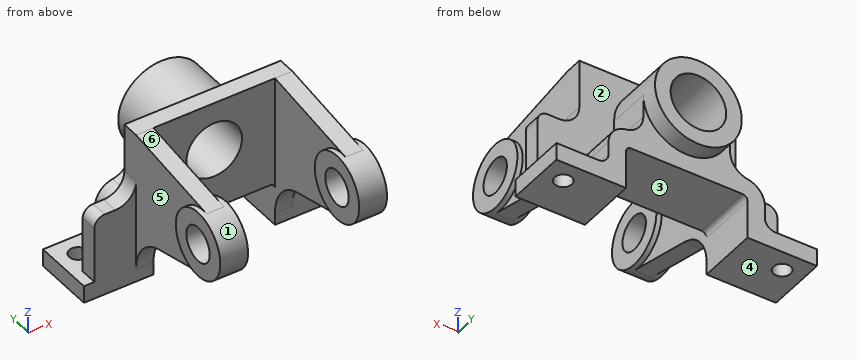
from build123d import *

# Parameters (mm, degrees)
BOSS_EXTRUDE1_DEPTH   = 10
SKETCH1_3_R           = 25
SKETCH1_3_R_2         = 16
BOSS_EXTRUDE2_DEPTH   = 45
BOSS_EXTRUDE3_DEPTH   = 35
FILLET1_R             = 12
BOSS_EXTRUDE4_DEPTH   = 10
BOSS_EXTRUDE5_START   = 3
SKETCH2_3_R           = 19
SKETCH2_3_R_2         = 10
BOSS_EXTRUDE5_DEPTH   = 16
FILLET2_R             = 25
MIRROR1_START         = -45
MIRROR1_OUTLINE_R     = 10
MIRROR1_DEPTH         = 10
MIRROR1_START_2       = -48
MIRROR1_2_OUTLINE_R   = 19
MIRROR1_2_OUTLINE_R_2 = 10
MIRROR1_2_DEPTH       = 16
SKETCH3_R             = 5
CUT_EXTRUDE1_DEPTH    = 133.483106346


# Read off the part's stored shape, not the designer's step: Mirror1
with BuildPart() as part:
    # Sketch1 → Boss-Extrude1 (new body)
    with BuildSketch(Plane(origin=(0, 0, 0), x_dir=(1, 0, 0), z_dir=(0, 1, 0))):
        with BuildLine():
            Line((-51, 50), (-69, 50))
            Line((-69, 50), (-69, 18))
            ThreePointArc((-69, 18), (-67.242640687, 13.757359313), (-63, 12))
            Line((-63, 12), (-57, 12))
            ThreePointArc((-57, 12), (-48.514718626, 8.485281374), (-45, 0))
            Line((-45, 0), (-45, -28))
            Line((-45, -28), (45, -28))
            Line((45, -28), (45, 0))
            ThreePointArc((45, 0), (48.514718626, 8.485281374), (57, 12))
            Line((57, 12), (63, 12))
            ThreePointArc((63, 12), (67.242640687, 13.757359313), (69, 18))
            Line((69, 18), (69, 50))
            Line((69, 50), (51, 50))
            ThreePointArc((51, 50), (46.757359313, 48.242640687), (45, 44))
            Line((45, 44), (45, 25))
            Line((45, 25), (37, 25))
            ThreePointArc((37, 25), (28.514718626, 21.485281374), (25, 13))
            Line((25, 13), (25, 0))
            ThreePointArc((25, 0), (0, -25), (-25, 0))
            Line((-25, 0), (-25, 13))
            ThreePointArc((-25, 13), (-28.514718626, 21.485281374), (-37, 25))
            Line((-37, 25), (-45, 25))
            Line((-45, 25), (-45, 44))
            ThreePointArc((-45, 44), (-46.757359313, 48.242640687), (-51, 50))
        make_face()
    extrude(amount=BOSS_EXTRUDE1_DEPTH)

    # Sketch1<3> → Boss-Extrude2 (add)
    with BuildSketch(Plane(origin=(0, 0, 0), x_dir=(1, 0, 0), z_dir=(0, 1, 0))):
        Circle(SKETCH1_3_R)
        with Locations(Location((0, 0, 0), (0, 0, 90))):
            Circle(SKETCH1_3_R_2, mode=Mode.SUBTRACT)
    extrude(amount=BOSS_EXTRUDE2_DEPTH)

    # Sketch1<4> → Boss-Extrude3 (add)
    with BuildSketch(Plane(origin=(0, 0, 0), x_dir=(1, 0, 0), z_dir=(0, 1, 0))):
        with BuildLine():
            Line((32, 35), (-32, 35))
            ThreePointArc((-32, 35), (-34.121320344, 35.878679656), (-35, 38))
            Line((-35, 38), (-35, 60))
            Line((-35, 60), (-75, 60))
            Line((-75, 60), (-75, 50))
            Line((-75, 50), (-69, 50))
            Line((-69, 50), (-51, 50))
            ThreePointArc((-51, 50), (-46.757359313, 48.242640687), (-45, 44))
            Line((-45, 44), (-45, 25))
            Line((-45, 25), (-37, 25))
            ThreePointArc((-37, 25), (-28.514718626, 21.485281374), (-25, 13))
            Line((-25, 13), (-25, 0))
            ThreePointArc((-25, 0), (0, 25), (25, 0))
            Line((25, 0), (25, 13))
            ThreePointArc((25, 13), (28.514718626, 21.485281374), (37, 25))
            Line((37, 25), (45, 25))
            Line((45, 25), (45, 44))
            ThreePointArc((45, 44), (46.757359313, 48.242640687), (51, 50))
            Line((51, 50), (69, 50))
            Line((69, 50), (75, 50))
            Line((75, 50), (75, 60))
            Line((75, 60), (35, 60))
            Line((35, 60), (35, 38))
            ThreePointArc((35, 38), (34.121320344, 35.878679656), (32, 35))
        make_face()
    extrude(amount=BOSS_EXTRUDE3_DEPTH)

    # Fillet1
    fillet1_edges = [part.edges().sort_by_distance(p)[0] for p in [
        (-45, 22.5, -25),
        (45, 22.5, -25),
    ]]
    fillet(fillet1_edges, radius=FILLET1_R)

    # Sketch2 → Boss-Extrude4 (add)
    with BuildSketch(Plane(origin=(45, 0, 0), x_dir=(0, 0, -1), z_dir=(1, 0, 0))):
        with BuildLine():
            Line((0, 0), (-28, 0))
            Line((-28, 0), (-18.781868567, -60.308822731))
            ThreePointArc((-18.781868567, -60.308822731), (-14.414314705, -45.059525702), (0, -38.438036581))
            Line((0, -38.438036581), (0, 0))
        make_face()
        with BuildLine():
            Line((33, 0), (0, 0))
            Line((0, 0), (0, -38.438036581))
            ThreePointArc((0, -38.438036581), (13.435028843, -44.003007739), (19, -57.438036581))
            ThreePointArc((19, -57.438036581), (18.873874635, -59.623638617), (18.497173025, -61.780223826))
            Line((18.497173025, -61.780223826), (33, 0))
        make_face()
    extrude(amount=-BOSS_EXTRUDE4_DEPTH)

    # Sketch2<3> → Boss-Extrude5 (add)
    with BuildSketch(Plane(origin=(45, 0, 0), x_dir=(0, 0, -1), z_dir=(1, 0, 0)).offset(BOSS_EXTRUDE5_START)):
        with Locations((0, -57.438036581)):
            Circle(SKETCH2_3_R)
        with Locations((0, -57.438036581)):
            Circle(SKETCH2_3_R_2, mode=Mode.SUBTRACT)
    extrude(amount=-BOSS_EXTRUDE5_DEPTH)

    # Fillet2
    # the kernel refuses this fillet: 25 mm, written as the material it adds along each edge
    with BuildSketch(Plane(origin=(45, 0, -33), x_dir=(0, 0, -1), z_dir=(-1, 0, 0))) as fillet2_piece_1:
        with BuildLine():
            CenterArc((FILLET2_R * 0.792435294557, FILLET2_R), FILLET2_R, 193.210905315, 76.789094685)
            Line((-FILLET2_R * 0.181100127826, FILLET2_R * 0.771463829198), (0, 0))
            Line((0, 0), (FILLET2_R * 0.792435294557, 0))
        make_face()
    extrude(amount=10)

    # Mirror1 outline → Mirror1 (add)
    with BuildSketch(Plane.YZ.offset(MIRROR1_START)):
        with BuildLine():
            Line((0, 28), (-60.308822731, 18.781868567))
            ThreePointArc((-60.308822731, 18.781868567), (-76.423254036, 0.74934517), (-61.780223826, -18.497173025))
            Line((-61.780223826, -18.497173025), (-19.28659573, -28.472496804))
            ThreePointArc((-19.28659573, -28.472496804), (-5.406185839, -37.284052468), (0, -52.810882364))
            Line((0, -52.810882364), (0, 28))
        make_face()
        with Locations((-57.438036581, 0)):
            Circle(MIRROR1_OUTLINE_R, mode=Mode.SUBTRACT)
    extrude(amount=MIRROR1_DEPTH)

    # Mirror1 2 outline → Mirror1 2 (add)
    with BuildSketch(Plane.YZ.offset(MIRROR1_START_2)):
        with Locations((-57.438036581, 0)):
            Circle(MIRROR1_2_OUTLINE_R)
        with Locations((-57.438036581, 0)):
            Circle(MIRROR1_2_OUTLINE_R_2, mode=Mode.SUBTRACT)
    extrude(amount=MIRROR1_2_DEPTH)

    # Sketch3 → Cut-Extrude1 (cut, through all)
    with BuildSketch(Plane.XY.offset(-50)):
        with Locations((63, 23)):
            Circle(SKETCH3_R)
    cut_extrude1 = extrude(amount=-CUT_EXTRUDE1_DEPTH, mode=Mode.SUBTRACT)

    # Mirror2: Cut-Extrude1 across plane
    add(cut_extrude1.mirror(Plane(origin=(0, 0, 0), x_dir=(0, 0, 1), z_dir=(1, 0, 0))), mode=Mode.SUBTRACT)


solid = part.part
Geometry check sheet. Reference: the model listing, model coordinates, mm. Face numbers are marked on the shaded views. A direction names the side the tool comes from. Round coordinates to 2 decimals unless told otherwise and drop trailing zeros. Order: outer loops, then holes, each group sorted by start corner. A loop starts at its lowest first (then second) coordinate and runs counter-clockwise, first axis right, second up. Notation, with made-up numbers: (50, 58) - (65, 58) arc R23 cw to (65, 83) - close; hole circle Ø8 at (70, -23). An arc over 180 degrees is marked (long way). One line per question, with ' | ' between items. Start each with the question number.
(1) Sectioned sample at C-C on z = 4. Count the separate pieces of the cut face and the enclosed holes in it, and give its area (3 significant figures).
(2) Release check for a two-part mould opening along Y. For the marked faces 4, 5 and 6 record: released by +Y, released by -Y, zero draft, split by the parting line, or undercut.
(3) Sectioned sample at B-B on y = 7. Record the cut outline in (x, z).
(4) Depth check by flat-ended pin: pin 1 Ø8 at (x, z) = (35, -6.5) entering from +Y; pin 2 Ø5 at (x, z) = (6.5, -36.5) entering from -Y; pin 3 Ø19 at (y, z) = (-61, -1) entering from +X; pin 4 Ø18 at (y, z) = (-57.44, 0) entering from -X. Enter the tip coordinate at first touch or a pass-through.
(5) Sectioned sample at A-A on x = 0. Record the cut outline in (y, z), and give its area (3 significant figures).
(6) Access from +Z, -Z, +X, -X, +Y, -Y to the whole of each face (thin tool, end or side, straight path). Record for the marked faces 1, 2 and 3.
(7) Thickness scan on L1, parallel to X at y = -22, z = 7.5; L2, parallel to Y at x = 63, z = -55.25; L3, parallel to Z at x = 1, y = 17.5. Record the ranges inside material, lowest first. Write a range as [from, to].
Conclusion:
1) separate pieces: 4 | enclosed holes: 0 | area: 2,610 mm2
2) face 4: zero draft | face 5: undercut | face 6: released by -Y
3) outline: (-75, -60) - (-35, -60) - (-35, -38) arc R3 cw to (-32, -35) - (32, -35) arc R3 cw to (35, -38) - (35, -60) - (75, -60) - (75, -50) - (69, -50) - (69, -18) arc R6 ccw to (63, -12) - (57, -12) arc R12 cw to (45, 0) - (45, 28) - (-45, 28) - (-45, 0) arc R12 cw to (-57, -12) - (-63, -12) arc R6 ccw to (-69, -18) - (-69, -50) - (-75, -50) - close; hole circle Ø32 at (0, 0)
4) pin 1: stops at y = 10 | pin 2: stops at y = 0 | pin 3: stops at x = 48 | pin 4: passes through
5) outline: (0, -35) - (35, -35) - (35, -25) - (45, -25) - (45, -16) - (0, -16) - close; (0, 16) - (45, 16) - (45, 25) - (10, 25) - (10, 28) - (0, 28) - close | area: 1,190 mm2
6) face 1: none | face 2: +Z, +Y | face 3: -Z, +Y, -Y
7) L1: x = [-45, -35], [35, 45] | L2: y = [0, 18], [28, 35] | L3: z = [-35, -15.97], [15.97, 24.98]
